The model under review builds one solid part; all positions refer to its coordinate system, in mm. A direction names the side the tool comes from. Round coordinates to 2 decimals unless told otherwise and drop trailing zeros. Order: outer loops, then holes, each group sorted by start corner. A loop starts at its lowest first (then second) coordinate and runs counter-clockwise, first axis right, second up. Notation, with made-up numbers: (-31.75, -30.5) -> (13.25, -30.5) arc R18 cw to (13.25, -5.5) -> close; hole circle Ø8 at (-34.5, 47.25). An arc over 180 degrees is marked (long way). Use a Markdown table: item, result. Add a question column.
```python
from build123d import *

# Parameters (mm, degrees)
BOSS_EXTRUDE1_DEPTH      = 2
BOSS_EXTRUDE1_DEPTH_BACK = 2
BOSS_EXTRUDE2_DEPTH      = 7.1
BOSS_EXTRUDE2_DEPTH_BACK = 7.1
SKETCH1_4_R              = 1.8


with BuildPart() as part:
    # Sketch1 → Boss-Extrude1 (new, two sides: drawn at the far end of the back side and taken through both)
    with BuildSketch(Plane(origin=(0, 0, 0), x_dir=(1, 0, 0), z_dir=(0, 1, 0)).offset(-BOSS_EXTRUDE1_DEPTH_BACK)):
        with BuildLine():
            ThreePointArc((-4.2, -9), (-4.727207794, -10.272792206), (-6, -10.8))
            Line((-6, -10.8), (6, -10.8))
            ThreePointArc((6, -10.8), (4.2, -9), (6, -7.2))
            Line((6, -7.2), (2, -7.2))
            Line((2, -7.2), (2, 7.2))
            Line((2, 7.2), (6, 7.2))
            ThreePointArc((6, 7.2), (4.2, 9), (6, 10.8))
            Line((6, 10.8), (-6, 10.8))
            ThreePointArc((-6, 10.8), (-4.727207794, 10.272792206), (-4.2, 9))
            ThreePointArc((-4.2, 9), (-4.727207794, 7.727207794), (-6, 7.2))
            Line((-6, 7.2), (-2, 7.2))
            Line((-2, 7.2), (-2, -7.2))
            Line((-2, -7.2), (-6, -7.2))
            ThreePointArc((-6, -7.2), (-4.727207794, -7.727207794), (-4.2, -9))
        make_face()
    extrude(amount=BOSS_EXTRUDE1_DEPTH + BOSS_EXTRUDE1_DEPTH_BACK)

    # Sketch1_4 → Boss-Extrude2 (add, two sides: drawn at the far end of the back side and taken through both)
    with BuildSketch(Plane(origin=(0, 0, 0), x_dir=(1, 0, 0), z_dir=(0, 1, 0)).offset(-BOSS_EXTRUDE2_DEPTH_BACK)):
        with Locations(Location((-6, 9, 0), (0, 0, 270))):
            Circle(SKETCH1_4_R)
        with Locations(Location((6, 9, 0), (0, 0, 270))):
            Circle(SKETCH1_4_R)
        with Locations(Location((-6, -9, 0), (0, 0, 270))):
            Circle(SKETCH1_4_R)
        with Locations(Location((6, -9, 0), (0, 0, 270))):
            Circle(SKETCH1_4_R)
    extrude(amount=BOSS_EXTRUDE2_DEPTH + BOSS_EXTRUDE2_DEPTH_BACK)


solid = part.part
```
Q1. Add section D-D (y = 0.25). Write out the cut boundary in (x, z).
Q2. Insertion check: pin 1 (2 mm diameter, centred on x = 1.5, z = 0.5, fed in from -Y); pin 2 (3 mm diameter, centred on y = 0, z = 3.5, fed in from +X); pin 3 (2 mm diameter, centred on y = 0.5, z = 3, fed in from -X). Each pin has a flat end and moves straight along its axis. Give the tip position at first contact, or say it passes through.
Q3. Mouldability with a two-part tool opening along X and no side actions: class faces 1 (the cylindrical face through (-7.757, -0.099, 8.61)), 2 (the flat face through (-2, 0, 0)), 3 (the flat face through (0, 2, 0)), 4 (the flat face through (-6, 7.1, 9)) as pulls with the +X half, pulls with the -X half, needs draft (parallel to the pull), parting line crosses it, or undercut.
Q4. Wall thickness on line 1 (Y direction, x = 1.25, z = -0.5); line 2 (Z direction, x = 6.75, y = 2.25): over which ranges is each line inside the solid? List them lowest first. Write a range as [from, to].
Q5. Add section C-C (z = -9). Write out the cut boundary in (x, y), then the cut area to 3 significant figures.
Q6. Machinability: for faces 5 (the flat face through (2, 0, 0)), 6 (the cylindrical face through (7.785, -0.099, -9.234)), 7 (the flat face through (-4, 0, -7.2)), 8 (the flat face through (6, 7.1, -9)), which of the approach directions +Z, -Z, +X, -X, +Y, -Y give a long, thin tool a straight path to every point of the face, cutting with its end or side? Answer none if there is none.
Q7. Add section B-B (y = 4.75). Write out the cut boundary in (x, z).
Q8. Add section A-A (x = 3.25). Write out the cut boundary in (y, z).
Report:
| question | item | result |
|---|---|---|
| 1 | outline | (-6, -10.8) -> (6, -10.8) arc R1.8 ccw to (6, -7.2) -> (2, -7.2) -> (2, 7.2) -> (6, 7.2) arc R1.8 ccw to (6, 10.8) -> (-6, 10.8) arc R1.8 ccw to (-6, 7.2) -> (-2, 7.2) -> (-2, -7.2) -> (-6, -7.2) arc R1.8 ccw to start |
| 2 | pin 1 | stops at y = -2 |
| 2 | pin 2 | stops at x = 2 |
| 2 | pin 3 | stops at x = -2 |
| 3 | face 1 | undercut |
| 3 | face 2 | pulls with the -X half |
| 3 | face 3 | undercut |
| 3 | face 4 | needs draft |
| 4 | line 1 | y = [-2, 2] |
| 4 | line 2 | z = [-10.64, -7.36], [7.36, 10.64] |
| 5 | outline | (-7.8, -7.1) -> (-4.2, -7.1) -> (-4.2, -2) -> (4.2, -2) -> (4.2, -7.1) -> (7.8, -7.1) -> (7.8, 7.1) -> (4.2, 7.1) -> (4.2, 2) -> (-4.2, 2) -> (-4.2, 7.1) -> (-7.8, 7.1) -> close |
| 5 | area | 136 mm² |
| 6 | face 5 | +X, +Y, -Y |
| 6 | face 6 | none |
| 6 | face 7 | -X, +Y, -Y |
| 6 | face 8 | +Z, -Z, +X, -X, +Y |
| 7 | outline | circle Ø3.6 at (-6, -9); circle Ø3.6 at (-6, 9); circle Ø3.6 at (6, -9); circle Ø3.6 at (6, 9) |
| 8 | outline | (-2, -10.8) -> (2, -10.8) -> (2, -7.2) -> (-2, -7.2) -> close; (-2, 7.2) -> (2, 7.2) -> (2, 10.8) -> (-2, 10.8) -> close |
